```python
from build123d import *

# Parameters (mm, degrees)
F0_R     = 38.7
F0_R_2   = 3
F0_R_3   = 1.5
F1_DEPTH = 2


# Not quite as in the source:
# - a fillet or chamfer that OpenCascade refuses, or shapes differently, is made with other operations: its cross-section is extruded or revolved along the edge and cut away or added


with BuildPart() as f1:
    # F0 (on Top) → F1 (new body)
    with BuildSketch(Plane.XY):
        Circle(F0_R)
        with Locations((0, -21.5)):
            Circle(F0_R_2, mode=Mode.SUBTRACT)
        with Locations((-21.5, 0)):
            Circle(F0_R_2, mode=Mode.SUBTRACT)
        Circle(F0_R_3, mode=Mode.SUBTRACT)
        with Locations((21.5, 0)):
            Circle(F0_R_2, mode=Mode.SUBTRACT)
        with Locations((0, 21.5)):
            Circle(F0_R_2, mode=Mode.SUBTRACT)
    extrude(amount=F1_DEPTH)

    # F2: fillet of radius 3 on 1 edges, made by hand

    # F2_s1 → F2_t2 (revolve, cut)
    with BuildSketch(Plane.XZ):
        with BuildLine():
            ThreePointArc((38.7, 0), (37.6036236828, 1.4494897428), (35.8715728753, 2))
            Line((35.8715728753, 2), (38.7, 2))
            Line((38.7, 2), (38.7, 0))
        make_face()
    revolve(axis=Axis((0, 0, 2), (0, 0, 1)), mode=Mode.SUBTRACT)


solid = f1.part
```
The model under review builds one solid part; all positions refer to its coordinate system, in mm. Round coordinates to 2 decimals unless told otherwise and drop trailing zeros. Order: outer loops, then holes, each group sorted by start corner. A loop starts at its lowest first (then second) coordinate and runs counter-clockwise, first axis right, second up. Notation, with made-up numbers: M -5.5,-11.75 L 46.5,-11.75 A31 cw 46.5,26.25 Z; hole C 45.5,59.25 d1. An arc over 180 degrees is marked long. Use a Markdown table: item, result.
1) Wall thickness on line 1 along Y through (x, z) = (0, 0.4); line 2 along Y through (x, z) = (0, 0.65); line 3 along Y through (x, z) = (-2, 1.2): over which ranges is each line inside the solid? List them lowest first. Write a range as [from, to].
Report:
| item | result |
|---|---|
| line 1 | [-38.52, -24.5], [-18.5, -1.5], [1.5, 18.5], [24.5, 38.52] |
| line 2 | [-38.38, -24.5], [-18.5, -1.5], [1.5, 18.5], [24.5, 38.38] |
| line 3 | [-37.86, -23.74], [-19.26, 19.26], [23.74, 37.86] |
2) Draft analysis for pull direction Y (two halves, no side actions). For faces 1 (the face through (-0.65, 18.57, 0.99)), 2 (the face through (-1, -8, 0)), state which applies: released by +Y, released by -Y, zero draft, split by the parting line, or undercut.
Report:
| item | result |
|---|---|
| face 1 | undercut |
| face 2 | zero draft |
3) Consider section A-A (y = 0). Write out the cut boundary in (x, z), then the cut area to 3 significant figures.
Report:
| item | result |
|---|---|
| outline | M -38.7,0 L -24.5,0 L -24.5,2 L -35.87,2 A3 ccw Z; M -18.5,0 L -1.5,0 L -1.5,2 L -18.5,2 Z; M 1.5,0 L 18.5,0 L 18.5,2 L 1.5,2 Z; M 24.5,0 L 38.7,0 A3 ccw 35.87,2 L 24.5,2 Z |
| area | 122 mm^2 |
4) Consider section C-C (z = 0.8). Write out the cut boundary in (x, y).
Report:
| item | result |
|---|---|
| outline | C 0,0 d76.54; hole C -21.5,0 d6; hole C 0,-21.5 d6; hole C 0,21.5 d6; hole C 0,0 d3; hole C 21.5,0 d6 |
